Model file for the job. Use its own axes, mm. Give positions to 0.01 mm unless a question says otherwise; leave off trailing zeros. Loops run counter-clockwise (first coordinate to the right, second up) from the corner with the lowest first, then second, coordinate; pieces in that order, holes last. Notation, with made-up numbers: (57, -9) - (92, -9) arc R14 ccw to (92, 5) - close; hole circle Ø4 at (-18.5, 56.5). An arc over 180 degrees is marked (long way). Answer as CSV lines item,"result". Start each with the question number.
Item 1: Drill centre line: L1, parallel to X at y = -3.5, z = 0.8. Where is it in solid material? Low to high. Write a range as from..to.
Item 2: Pin check, flat tips, straight feed: pin 1 (5 mm diameter, centred on x = -24.5, y = -2, fed in from -Z); pin 2 (1.5 mm diameter, centred on y = 3.5, z = 1, fed in from -X). Stop position of each tip, or through.
Item 3: Saw through at B-B on y = -6. Give the cut face in (x, z).
Item 4: Saw through at A-A on z = 2.2. Give the cut face in (x, y), plus the area to 3 significant figures.
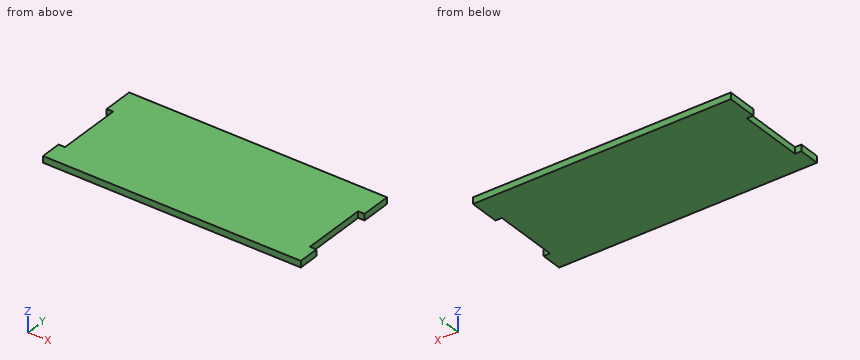
Autodesk Inventor part; units mm, degrees
ref_plane "YZ Plane" through (0, 0, 0) normal (1, 0, 0) x (0, 1, 0)
ref_plane "XZ Plane" through (0, 0, 0) normal (0, 1, 0) x (-1, 0, 0)
ref_plane "XY Plane" through (0, 0, 0) normal (0, 0, 1) x (1, 0, 0)
sketch "Esboço1" plane through (0, 0, 0) normal (0, 0, 1) x (1, 0, 0)
  line L0 (60, -27) -> (-60, -27)
  line L1 (-60, -27) -> (-60, 27)
  line L2 (-60, 27) -> (60, 27)
  line L3 (60, 27) -> (60, -27)
  line L4 (60, -27) -> (-60, 27) construction
  line L5 (-60, -27) -> (60, 27) construction
  point P0 (0, 0)
  dimension "d0" = 120
  dimension "d1" = 54
extrude "Extrusão1" add sketch "Esboço1" along normal blind 3
sketch "Esboço2" plane through (60, -27, 0) normal (1, 0, 0) x (0, 0, -1)
  line L0 (0, 54) -> (0, 43.9)
  line L1 (0, 54) -> (0, 0)
  line L2 (0, 0) -> (0, 9.75)
  line L3 (0, 9.75) -> (-3, 9.75)
  line L4 (-3, 9.75) -> (-3, 39.95)
  line L5 (-3, 39.95) -> (0, 39.95)
  line L6 (0, 39.95) -> (0, 9.75)
  point P0 (0, 27)
  point P1 (0, 39.95)
  point P2 (-1.5, 9.75)
  point P3 (-1.5, 39.95)
  dimension "d5" = 9.75
  dimension "d6" = 3
  dimension "d22" = 30.2
extrude "Extrusão2" cut sketch "Esboço2" against normal blind 3
sketch "Esboço3" plane through (-60, -27, 0) normal (-1, 0, 0) x (0, 0, 1)
  line L0 (3, 39.95) -> (3, 54)
  line L1 (3, 54) -> (3, 39.95)
  line L2 (3, 0) -> (3, 9.75)
  line L3 (3, 0) -> (3, 9.75)
  line L4 (0, 39.95) -> (0, 9.75)
  line L5 (3, 9.75) -> (0, 9.75)
  line L6 (0, 9.75) -> (0, 39.95)
  line L7 (0, 39.95) -> (3, 39.95)
  line L8 (3, 39.95) -> (3, 9.75)
  point P0 (0, 27)
extrude "Extrusão3" cut sketch "Esboço3" against normal blind 3
sketch "Esboço4" plane through (-60, 27, 0) normal (0, 1, 0) x (1, 0, 0)
  point P0 (60, 0)
properties part number "top inclinado"
Responses:
1,L1,"-57..57"
2,pin 1,"z = 0"
2,pin 2,"x = -57"
3,outline,"(-57, 0) - (57, 0) - (57, 3) - (-57, 3) - close"
4,outline,"(-60, -27) - (60, -27) - (60, -17.25) - (57, -17.25) - (57, 12.95) - (60, 12.95) - (60, 27) - (-60, 27) - (-60, 12.95) - (-57, 12.95) - (-57, -17.25) - (-60, -17.25) - close"
4,area,"6,300 mm2"
